Model file for the job. Use its own axes, mm. Face numbers are marked on the shaded views. A direction names the side the tool comes from. Round coordinates to 2 decimals unless told otherwise and drop trailing zeros. Order: outer loops, then holes, each group sorted by start corner. A loop starts at its lowest first (then second) coordinate and runs counter-clockwise, first axis right, second up. Notation, with made-up numbers: (41, -16) - (85, -16) arc R27 cw to (85, 20) - close; hole circle Ø5 at (29.25, -11.5). An arc over 180 degrees is marked (long way). Use one line per item in the form item = value.
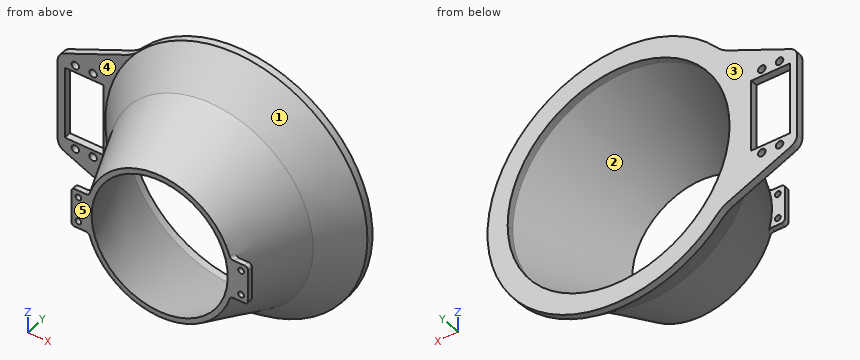
from build123d import *

# Parameters (mm, degrees)
SKETCH3_R           = 1.65
BOSS_EXTRUDE1_DEPTH = 3
FILLET1_R           = 2
SKETCH4_R           = 2.125
SKETCH4_W           = 22
SKETCH4_H           = 41
BOSS_EXTRUDE2_DEPTH = 4
BOSS_EXTRUDE3_DEPTH = 4
FILLET4_R           = 20
FILLET5_R           = 6


with BuildPart() as part:
    # Sketch2 → Revolve1 (revolve)
    with BuildSketch(Plane.XY, mode=Mode.PRIVATE) as revolve1_sk:
        Polygon((38.5, 0), (62.74157355, 60), (66.137606882, 60), (41.5, 0), align=None)
    revolve(revolve1_sk.sketch.rotate(Axis((0, 0, 0), (0, 1, 0)), 90), axis=Axis((0, 0, 0), (0, 1, 0)))

    # Sketch3 → Boss-Extrude1 (add)
    # profile 1 of 2: a face of its own
    with BuildSketch(Plane.XZ):
        with BuildLine():
            Line((-50.015621949, 11), (-40.015621949, 11))
            ThreePointArc((-40.015621949, 11), (-41.5, 0), (-40.015621949, -11))
            Line((-40.015621949, -11), (-50.015621949, -11))
            Line((-50.015621949, -11), (-50.015621949, 11))
        make_face()
        with Locations(Location((-46.015621949, -7, 0), (0, 0, 270))):
            Circle(SKETCH3_R, mode=Mode.SUBTRACT)
        with Locations(Location((-46.015621949, 7, 0), (0, 0, 90))):
            Circle(SKETCH3_R, mode=Mode.SUBTRACT)
    # profile 2 of 2: a face of its own
    with BuildSketch(Plane.XZ):
        with BuildLine():
            Line((50.015621949, -11), (40.015621949, -11))
            ThreePointArc((40.015621949, -11), (41.5, 0), (40.015621949, 11))
            Line((40.015621949, 11), (50.015621949, 11))
            Line((50.015621949, 11), (50.015621949, -11))
        make_face()
        with Locations(Location((46.015621949, 7, 0), (0, 0, 270))):
            Circle(SKETCH3_R, mode=Mode.SUBTRACT)
        with Locations(Location((46.015621949, -7, 0), (0, 0, 90))):
            Circle(SKETCH3_R, mode=Mode.SUBTRACT)
    extrude(amount=-BOSS_EXTRUDE1_DEPTH)

    # Fillet1
    fillet1_edges = [part.edges().sort_by_distance(p)[0] for p in [
        (-40.654005454, 1.499876919, -11),
        (-40.654005454, 1.499876919, 11),
        (-50.015621949, 1.5, -11),
        (-50.015621949, 1.5, 11),
        (40.654005454, 1.499876919, -11),
        (40.654005454, 1.499876919, 11),
        (50.015621949, 1.5, 11),
        (50.015621949, 1.5, -11),
    ]]
    fillet(fillet1_edges, radius=FILLET1_R)



with BuildPart() as body_2:
    # Sketch4 → Boss-Extrude2 (new body)
    with BuildSketch(Plane(origin=(0, 60, 0), x_dir=(1, 0, 0), z_dir=(0, 1, 0))):
        with BuildLine():
            Line((-33.439731634, 57.061084746), (-101, 27))
            Line((-101, 27), (-101, -27))
            Line((-101, -27), (-33.439731634, -57.061084746))
            Line((-33.439731634, -57.061084746), (-20, -63.04112185))
            ThreePointArc((-20, -63.04112185), (66.137606882, 0), (-20, 63.04112185))
            Line((-20, 63.04112185), (-33.439731634, 57.061084746))
        make_face()
        with Locations(Location((-91, -24.5, 0), (0, 0, 270))):
            Circle(SKETCH4_R, mode=Mode.SUBTRACT)
        with Locations(Location((-81, -24.5, 0), (0, 0, 270))):
            Circle(SKETCH4_R, mode=Mode.SUBTRACT)
        with Locations((-86, 0)):
            Rectangle(SKETCH4_W, SKETCH4_H, mode=Mode.SUBTRACT)
        with Locations(Location((-91, 24.5, 0), (0, 0, 270))):
            Circle(SKETCH4_R, mode=Mode.SUBTRACT)
        with Locations(Location((-81, 24.5, 0), (0, 0, 270))):
            Circle(SKETCH4_R, mode=Mode.SUBTRACT)
        with BuildLine():
            ThreePointArc((62.74157355, 0), (36.617438336, -50.947701236), (-20, -59.468521518))
            ThreePointArc((-20, -59.468521518), (-36.617438336, 50.947701236), (62.74157355, 0))
        make_face(mode=Mode.SUBTRACT)
    extrude(amount=BOSS_EXTRUDE2_DEPTH)


with BuildPart() as part_1:
    add(part.part)

    add(body_2.part)  # Revolve5 merges body 2
    # Sketch6 → Revolve5 (revolve)
    with BuildSketch(Plane.XY, mode=Mode.PRIVATE) as revolve5_sk:
        Polygon((-66.137606882, 60), (-74.137606882, 60), (-57.925071255, 40), align=None)
    revolve(revolve5_sk.sketch.rotate(Axis((0, 0, 0), (0, 1, 0)), 162.54936445), axis=Axis((0, 0, 0), (0, 1, 0)))

    # Sketch7 → Boss-Extrude3 (add)
    with BuildSketch(Plane(origin=(0, 60, 0), x_dir=(1, 0, 0), z_dir=(0, 1, 0))):
        with BuildLine():
            Line((-58.055144228, 46.108404688), (-20, 63.04112185))
            ThreePointArc((-20, 63.04112185), (66.137606882, 0), (-20, -63.04112185))
            Line((-20, -63.04112185), (-58.055144228, -46.108404688))
            ThreePointArc((-58.055144228, -46.108404688), (74.137606882, 0), (-58.055144228, 46.108404688))
        make_face()
    extrude(amount=BOSS_EXTRUDE3_DEPTH)

    # Fillet4
    fillet4_edges = [part_1.edges().sort_by_distance(p)[0] for p in [
        (-58.055144228, 62, 46.108404688),
        (-58.055144228, 62, -46.108404688),
    ]]
    fillet(fillet4_edges, radius=FILLET4_R)

    # Fillet5
    fillet5_edges = [part_1.edges().sort_by_distance(p)[0] for p in [
        (-101, 62, -27),
        (-101, 62, 27),
    ]]
    fillet(fillet5_edges, radius=FILLET5_R)


solid = part_1.part
(1) Tool access for the marked faces 4 and 5: list every direction of +Z, -Z, +X, -X, +Y, -Y with a clear straight run to the whole face (end or side of a thin tool).
Report:
face_4 = -X, -Y
face_5 = +Z, -Z, +X, -X, -Y
(2) Slice it at A-A on x = -91. Give the cut face in (y, z) (3 decimals), then the cut area to 3 significant figures.
Report:
outline = (60, -31.45) - (64, -31.45) - (64, -26.625) - (60, -26.625) - close; (60, -22.375) - (64, -22.375) - (64, -20.5) - (60, -20.5) - close; (60, 20.5) - (64, 20.5) - (64, 22.375) - (60, 22.375) - close; (60, 26.625) - (64, 26.625) - (64, 31.45) - (60, 31.45) - close
area = 53.6 mm2
(3) Pin check, flat tips, straight feed: pin 1 (1.5 mm diameter, centred on x = 45.5, y = 1, fed in from +Z); pin 2 (2 mm diameter, centred on x = -46.02, z = -7, fed in from +Y); pin 3 (2.5 mm diameter, centred on y = 1, z = 2.5, fed in from -X). Stop position of each tip, or through.
Report:
pin_1 = 11
pin_2 = 22.4
pin_3 = -50.02
(4) Pull direction X, two halves, no side cores. Call the marked faces 1, 2 and 3: released by +X, released by -X, zero draft, split by the parting line, or undercut.
Report:
face_1 = split by the parting line
face_2 = undercut
face_3 = zero draft
(5) Slice it at B-B on y = 30. Give the cut face in (x, z), then the cut area to 3 significant figures.
Report:
outline = circle Ø107.64 at (0, 0); hole circle Ø101.24 at (0, 0)
area = 1,050 mm2
(6) Probe probe 1 along X at (y, z) = (1.2, -7); probe 2 along X at (y, z) = (2, -7); probe 3 along Z at (x, y) = (30.5, 23). List the from-to ranges inside material, lowest first. Write a range as [from, to].
Report:
probe_1 = [-50.02, -47.67], [-44.37, -38.35], [38.35, 44.37], [47.67, 50.02]
probe_2 = [-50.02, -47.67], [-44.37, -38.68], [38.68, 44.37], [47.67, 50.02]
probe_3 = [-40.81, -36.8], [36.8, 40.81]
(7) Slice it at C-C on y = 11. Give the cut face in (x, z).
Report:
outline = circle Ø92.03 at (0, 0); hole circle Ø85.89 at (0, 0)
